Design review of the part shown in the three views and the two pictorial views. Dimensions are in mm from the part's minimum x, y and z. A direction names the side the tool comes from. Round coordinates to 2 decimals unless told otherwise and drop trailing zeros. Order: outer loops, then holes, each group sorted by start corner. A loop starts at its lowest first (then second) coordinate and runs counter-clockwise, first axis right, second up.
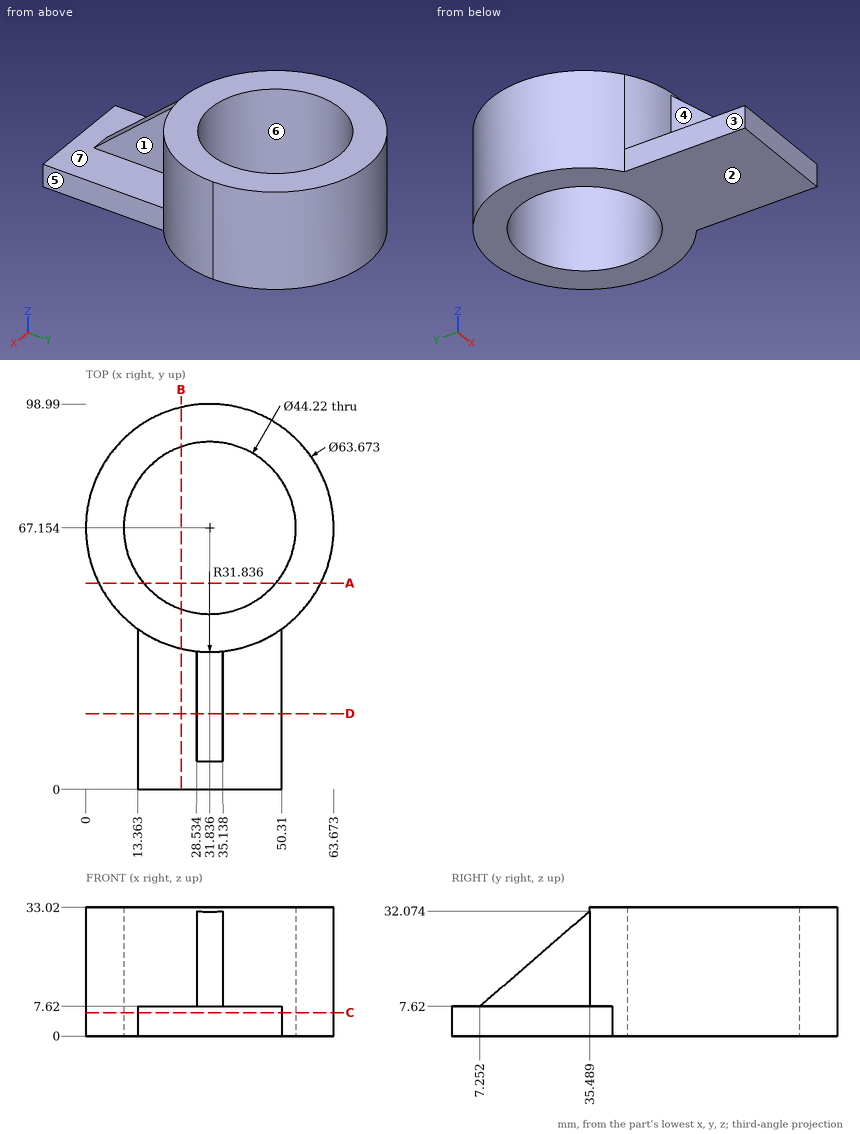
(1) Clearance check with flat-ended pins moving along their axes: P1, Ø4, axis at x = 8.5, z = 9, coming from the -Y side (1 decimal); P2, Ø6, axis at y = 43, z = 5, coming from the +X side; P3, Ø2, axis at y = 71.5, z = 23, coming from the -X side. State where each tip first meets the part, or that it passes through.
(2) Tool access review of the marked faces 1, 2 and 3: name each direction out of +Z, -Z, +X, -X, +Y, -Y from which nothing blocks a thin tool from reaching the whole face with its end or side.
(3) Add section C-C on z = 6. Give the boundary of the cut face in (x, y) (1 decimal).
(4) Add section B-B on x = 24.5. Give the boundary of the cut face in (y, z) (1 decimal).
(5) Draft analysis for pull direction X (two halves, no side actions). For the marked faces 4, 5, 6 and 7, state which applies: pulls with the +X half, pulls with the -X half, needs draft (parallel to the pull), parting line crosses it, or undercut.
(6) Add section A-A on y = 53. Give the boundary of the cut face in (x, z).
(7) Add section D-D on y = 19.5. Give the boundary of the cut face in (x, z) (1 decimal).
(8) Wall thickness on L1, parallel to X at y = 61.5, z = 30 (1 decimal); L2, parallel to X at y = 60, z = 11 (1 decimal); L3, parallel to Y at x = 16.5, z = 17.5 (1 decimal): over which ranges is each line inside the solid? List them lowest first.
Here are the results:
1. P1: stops at y = 43.5
1. P2: stops at x = 55.63
1. P3: stops at x = 0.18
2. face 1: +Z, +X, -Y
2. face 2: -Z, +X, -X, +Y, -Y
2. face 3: +Z, -Z, -X, -Y
3. outline: (13.4, 0) - (50.3, 0) - (50.3, 41.2) arc R31.8 ccw to (63.7, 67.2) arc R31.8 ccw (long way) to (13.4, 41.2) - close; hole circle Ø44.2 at (31.8, 67.2)
4. outline: (0, 0) - (46.3, 0) - (46.3, 33) - (36.2, 33) - (36.2, 7.6) - (0, 7.6) - close; (88, 0) - (98.1, 0) - (98.1, 33) - (88, 33) - close
5. face 4: pulls with the -X half
5. face 5: pulls with the +X half
5. face 6: undercut
5. face 7: needs draft
6. outline: (3.32, 0) - (14.85, 0) - (14.85, 33.02) - (3.32, 33.02) - close; (48.82, 0) - (60.35, 0) - (60.35, 33.02) - (48.82, 33.02) - close
7. outline: (13.4, 0) - (50.3, 0) - (50.3, 7.6) - (35.1, 7.6) - (35.1, 18.2) - (28.5, 18.2) - (28.5, 7.6) - (13.4, 7.6) - close
8. L1: x = 0.5 to 10.5, 53.2 to 63.2
8. L2: x = 0.8 to 10.9, 52.8 to 62.9
8. L3: y = 39.3 to 51.2, 83.1 to 95.1
